from build123d import *

# Parameters (mm, degrees)
SKETCH1_R           = 12.5
BOSS_EXTRUDE2_DEPTH = 10
CUT_EXTRUDE1_REACH  = 28.693
CHAMFER1_SIZE       = 1.5


with BuildPart() as part:
    # Sketch1 → Boss-Extrude2 (new body)
    with BuildSketch(Plane(origin=(0, 0, 0), x_dir=(1, 0, 0), z_dir=(0, 1, 0))):
        with Locations(Location((0, 0, 0), (0, 0, 270))):
            Circle(SKETCH1_R)
    extrude(amount=BOSS_EXTRUDE2_DEPTH)

    # Sketch2 → Revolve1 (revolve)
    with BuildSketch(Plane.XY):
        Polygon((5, 10), (0, 20), (0, 10), align=None)
    revolve(axis=Axis((0, -1000, 0), (0, 1, 0)))

    # Sketch3 → Cut-Extrude1 (cut, up to next)
    with BuildSketch(Plane(origin=(0, 0, 0), x_dir=(1, 0, 0), z_dir=(0, 1, 0)), mode=Mode.PRIVATE) as cut_extrude1_sk1:
        with BuildLine():
            Line((-10, 7.5), (-10, -7.5))
            ThreePointArc((-10, -7.5), (-12.5, 0), (-10, 7.5))
        make_face()
    cut_extrude1_tool1 = extrude(cut_extrude1_sk1.sketch, amount=CUT_EXTRUDE1_REACH, mode=Mode.PRIVATE) & part.part
    # Sketch3 → Cut-Extrude1 (cut, up to next)
    with BuildSketch(Plane(origin=(0, 0, 0), x_dir=(1, 0, 0), z_dir=(0, 1, 0)), mode=Mode.PRIVATE) as cut_extrude1_sk2:
        with BuildLine():
            Line((10, 7.5), (10, -7.5))
            ThreePointArc((10, -7.5), (12.5, 0), (10, 7.5))
        make_face()
    cut_extrude1_tool2 = extrude(cut_extrude1_sk2.sketch, amount=CUT_EXTRUDE1_REACH, mode=Mode.PRIVATE) & part.part
    add(cut_extrude1_tool1.solids().sort_by_distance((-11.0091, 0, 0))[0], mode=Mode.SUBTRACT)
    add(cut_extrude1_tool2.solids().sort_by_distance((11.0091, 0, 0))[0], mode=Mode.SUBTRACT)

    # Chamfer1
    chamfer1_edges = [part.edges().sort_by_distance(p)[0] for p in [
        (0, 10, -12.5),
        (0, 10, 12.5),
        (-10, 0, 0),
        (-10, 10, 0),
        (10, 0, 0),
        (10, 10, 0),
        (0, 0, -12.5),
        (0, 0, 12.5),
    ]]
    chamfer(chamfer1_edges, length=CHAMFER1_SIZE)


solid = part.part
Input: part model. Units: mm. Frame: model coordinates. A direction names the side the tool comes from. Coordinates: 2 decimals unless noted, no trailing zeros. Loops run counter-clockwise (first coordinate to the right, second up) from the corner with the lowest first, then second, coordinate; pieces in that order, holes last. Notation, with made-up numbers: (60.5, 66) -> (75.5, 66) arc R24 cw to (75.5, 103) -> close; hole circle Ø10 at (-13, 8). An arc over 180 degrees is marked (long way). One line per item, written item: value.
(1) Cut plane A-A (y = 13.75). Output: boundary loops of the cut face in (x, z) (3 decimals).
Answer below:
outline: circle Ø6.25 at (0, 0)
(2) Cut plane B-B (y = 16.75). Output: boundary loops of the cut face in (x, z) (3 decimals).
Answer below:
outline: circle Ø3.25 at (0, 0)
(3) Set-up query: faces 1 (the face through (-2, 10, -5)), 2 (the face through (-0.1, 0.2, 11.2)). Return all of +Z, -Z, +X, -X, +Y, -Y with unobstructed straight access to the full face (end or side cutting, diameter ignored); none if empty.
Answer below:
face 1: +Y
face 2: +Z, -Y
(4) Ray query, line 1 along Y through (x, z) = (3.25, 6.5); line 2 along Y through (x, z) = (0.5, 1.75); line 3 along X through (y, z) = (2, 9). Return the intervals inside material, ascending.
Answer below:
line 1: y = 0 to 10
line 2: y = 0 to 16.36
line 3: x = -8.67 to 8.67
(5) Pin query (flat end, axial travel): pin 1 Ø1.5 at (x, z) = (7.5, -5) entering from +Y; pin 2 Ø2 at (x, y) = (2, 10) entering from -Z; pin 3 Ø8 at (x, z) = (7, -3) entering from +Y. Return the tip coordinate at first contact, or that it passes through.
Answer below:
pin 1: stops at y = 10
pin 2: stops at z = -11.85
pin 3: stops at y = 12.77
